```python
from build123d import *

# Parameters (mm, degrees)
SKETCH_1_R          = 3
EXTRUDE_1_DEPTH     = 3
SKETCH_2_R          = 2
EXTRUDE_2_DEPTH     = 18
SKETCH_4_W          = 1
SKETCH_4_H          = 4.937645572
CUT_EXTRUDE_1_DEPTH = 6
FILLET_1_R          = 0.2


with BuildPart() as part:
    # 草图1 → 凸台-拉伸1 (new body)
    with BuildSketch(Plane(origin=(0, 0, 0), x_dir=(1, 0, 0), z_dir=(0, 1, 0))):
        with Locations(Location((0, 0, 0), (0, 0, 270))):
            Circle(SKETCH_1_R)
    extrude(amount=EXTRUDE_1_DEPTH)

    # 草图2 → 凸台-拉伸2 (add)
    with BuildSketch(Plane(origin=(0, 3, 0), x_dir=(1, 0, 0), z_dir=(0, 1, 0))):
        with Locations(Location((0, 0, 0), (0, 0, 270))):
            Circle(SKETCH_2_R)
    extrude(amount=EXTRUDE_2_DEPTH)

    # 草图3 → 旋转1 (revolve)
    with BuildSketch(Plane.XY, mode=Mode.PRIVATE) as revolve_1_sk:
        Polygon((0, 21), (-2, 21), (-2.1, 20), (0, 20), align=None)
    revolve(revolve_1_sk.sketch.rotate(Axis((0, 20, 0), (0, 1, 0)), 90), axis=Axis((0, 20, 0), (0, 1, 0)))

    # 草图4 → 切除-拉伸1 (cut)
    with BuildSketch(Plane(origin=(0, 21, 0), x_dir=(1, 0, 0), z_dir=(0, 1, 0))):
        Rectangle(SKETCH_4_W, SKETCH_4_H)
    extrude(amount=-CUT_EXTRUDE_1_DEPTH, mode=Mode.SUBTRACT)

    # 圆角1
    fillet_1_edges = [part.edges().sort_by_distance(p)[0] for p in [
        (0, 0, -3),
        (0, 3, -3),
    ]]
    fillet(fillet_1_edges, radius=FILLET_1_R)


solid = part.part
```
Part model, mm, in its own coordinate system. A direction names the side the tool comes from. Give positions to 0.01 mm unless a question says otherwise; leave off trailing zeros. Write each loop counter-clockwise with the first axis right and the second up, starting at its lowest first coordinate (ties: lowest second). Pieces come first, ordered by that corner, then holes. Notation, with made-up numbers: (-35.75, -31) -> (16.25, -31) arc R20 ccw to (16.25, -14) -> close; hole circle Ø2 at (-1.75, -5). An arc over 180 degrees is marked (long way). Put each result on its own line as item: value. Start each with the question number.
Item 1: Pin check, flat tips, straight feed: pin 1 Ø1 at (x, y) = (-1.5, 17) entering from +Z; pin 2 Ø2 at (x, y) = (2.5, 6.5) entering from +Z; pin 3 Ø2 at (y, z) = (3, -1.5) entering from -X. Stop position of each tip, or through.
Item 2: Wall check: L1, parallel to Y at x = 2, z = -1; L2, parallel to Z at x = 0, y = 12.5; L3, parallel to Y at x = -0.25, z = -1. Give the ranges that are in metal, low to high. Write a range as [from, to].
Item 3: Cut at B-B (y = 15.75). List the corners of the cut face in (x, z), then the cut area to 3 significant figures.
Item 4: Cut at C-C (z = 0). List the corners of the cut face in (x, y).
Item 5: Cut at A-A (x = 0). List the corners of the cut face in (y, z).
Item 6: Pull direction Y, two halves, no side cores. Call faces 1 (the face through (1, 21, 0)), 2 (the face through (0.9, 1.48, 2.86)), 3 (the face through (-0.766, 11.381, 1.847)), 4 (the face through (0, 0, 0)): pulls with the +Y half, pulls with the -Y half, needs draft (parallel to the pull), parting line crosses it, or undercut.
Item 7: Which spindle directions (+Z, -Z, +X, -X, +Y, -Y) get a long thin tool onto all of the face, cutting with end or side? Do faces 5 (the face through (0, 15, 0)), 6 (the face through (-1, 21, 0)). Say none if no direction does.
Item 8: Cut at D-D (y = 12.5). List the corners of the cut face in (x, z).
Answer list:
1. pin 1: stops at z = 1.73
1. pin 2: stops at z = 1.32
1. pin 3: stops at x = -2.95
2. L1: y = [0, 3]
2. L2: z = [-2, 2]
2. L3: y = [0, 15]
3. outline: (-0.5, -1.94) -> (-0.5, 1.94) arc R2 ccw to start; (0.5, -1.94) arc R2 ccw to (0.5, 1.94) -> close
3. area: 8.61 mm2
4. outline: (-3, 0.2) arc R0.2 ccw to (-2.8, 0) -> (2.8, 0) arc R0.2 ccw to (3, 0.2) -> (3, 2.8) arc R0.2 ccw to (2.8, 3) -> (2, 3) -> (2, 20) -> (2.1, 20) -> (2, 21) -> (0.5, 21) -> (0.5, 15) -> (-0.5, 15) -> (-0.5, 21) -> (-2, 21) -> (-2.1, 20) -> (-2, 20) -> (-2, 3) -> (-2.8, 3) arc R0.2 ccw to (-3, 2.8) -> close
5. outline: (0, -2.8) arc R0.2 ccw to (0.2, -3) -> (2.8, -3) arc R0.2 ccw to (3, -2.8) -> (3, -2) -> (15, -2) -> (15, 2) -> (3, 2) -> (3, 2.8) arc R0.2 ccw to (2.8, 3) -> (0.2, 3) arc R0.2 ccw to (0, 2.8) -> close
6. face 1: pulls with the +Y half
6. face 2: needs draft
6. face 3: undercut
6. face 4: pulls with the -Y half
7. face 5: +Z, -Z, +Y
7. face 6: +Z, -Z, +X, -X, +Y
8. outline: circle Ø4 at (0, 0)
